```python
from build123d import *

# Parameters (mm, degrees)
BASIS_BLECH1_DEPTH = 260
VERRUNDUNG1_R      = 10


# Sheet-metal steps are written as plain solids
with BuildPart() as part:
    # Skizze1 → Basis-Blech1 (new body)
    with BuildSketch(Plane.XY):
        with BuildLine():
            Line((-142, 50), (-142, 0.7366))
            ThreePointArc((-142, 0.7366), (-141.784254855, 0.215745145), (-141.2634, 0))
            Line((-141.2634, 0), (-0.7366, 0))
            ThreePointArc((-0.7366, 0), (-0.215745145, 0.215745145), (0, 0.7366))
            Line((0, 0.7366), (0, 50))
            Line((0, 50), (2, 50))
            Line((2, 50), (2, 0.7366))
            ThreePointArc((2, 0.7366), (1.198468417, -1.198468417), (-0.7366, -2))
            Line((-0.7366, -2), (-141.2634, -2))
            ThreePointArc((-141.2634, -2), (-143.198468417, -1.198468417), (-144, 0.7366))
            Line((-144, 0.7366), (-144, 50))
            Line((-144, 50), (-142, 50))
        make_face()
    extrude(amount=BASIS_BLECH1_DEPTH)

    # Verrundung1
    verrundung1_edges = [part.edges().sort_by_distance(p)[0] for p in [
        (-143, 50, 0),
        (1, 50, 0),
        (-143, 50, 260),
        (1, 50, 260),
    ]]
    fillet(verrundung1_edges, radius=VERRUNDUNG1_R)


solid = part.part
```
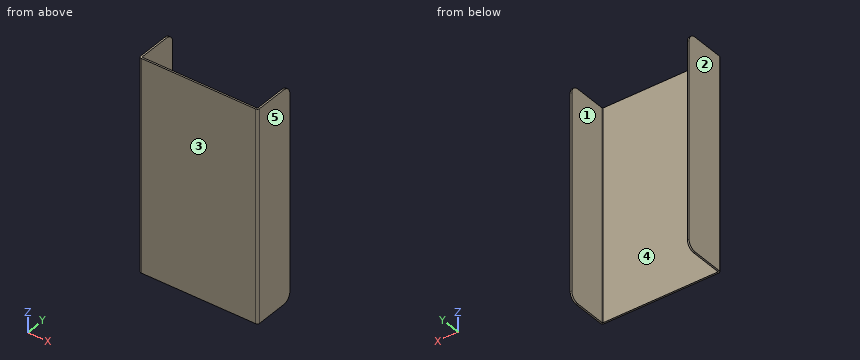
Check sheet for the modelled part. Datum: model origin and axes. Units: mm. Face numbers are marked on the shaded views. A direction names the side the tool comes from. Round coordinates to 2 decimals unless told otherwise and drop trailing zeros. Order: outer loops, then holes, each group sorted by start corner. A loop starts at its lowest first (then second) coordinate and runs counter-clockwise, first axis right, second up. Notation, with made-up numbers: (-7, -32.75) - (46, -32.75) arc R9 cw to (46, -21.75) - close; hole circle Ø9 at (79, 9.5). An arc over 180 degrees is marked (long way). Answer as CSV lines item,"result". Start each with the question number.
1) Tool access check on the marked faces 4 and 5. Record the directions out of +Z, -Z, +X, -X, +Y, -Y that give a thin tool (end or side, any length) a straight path to the whole face; none if there is none.
2) Scan lines: probe 1 along X at (y, z) = (5, 33.5); probe 2 along Y at (x, z) = (-63.5, 17). Record each from-to range of solid material in increasing order.
3) Section check A-A (y = 31). Record the cut outline in (x, z).
4) Section check D-D (y = 43.5). Record the cut outline in (x, z).
5) Depth check by flat-ended pin: pin 1 (2 mm diameter, centred on x = -58, z = 43.5, fed in from +Y). Enter the tip coordinate at first touch or a pass-through.
6) Section check B-B (z = 38). Record the cut outline in (x, y), then the cut area to 3 significant figures.
7) Draft check along X on the marked faces 1, 2 and 3. Enter one of: +X half, -X half, draft (parallel to the pull), parting line (faces both ways), or undercut.
8) Section check C-C (x = -66). Record the cut outline in (y, z).
Determined:
1,face 4,"+Z, -Z, +Y"
1,face 5,"+Z, -Z, +X, +Y, -Y"
2,probe 1,"-144 to -142, 0 to 2"
2,probe 2,"-2 to 0"
3,outline,"(-144, 0) - (-142, 0) - (-142, 260) - (-144, 260) - close; (0, 0) - (2, 0) - (2, 260) - (0, 260) - close"
4,outline,"(-144, 0.63) - (-142, 0.63) - (-142, 259.37) - (-144, 259.37) - close; (0, 0.63) - (2, 0.63) - (2, 259.37) - (0, 259.37) - close"
5,pin 1,"y = 0"
6,outline,"(-144, 0.74) arc R2.74 ccw to (-141.26, -2) - (-0.74, -2) arc R2.74 ccw to (2, 0.74) - (2, 50) - (0, 50) - (0, 0.74) arc R0.74 cw to (-0.74, 0) - (-141.26, 0) arc R0.74 cw to (-142, 0.74) - (-142, 50) - (-144, 50) - close"
6,area,"489 mm^2"
7,face 1,"undercut"
7,face 2,"-X half"
7,face 3,"draft"
8,outline,"(-2, 0) - (0, 0) - (0, 260) - (-2, 260) - close"
